The listing builds one solid part. Answer for the finished solid, in the listing's coordinates (mm). A direction names the side the tool comes from. Round coordinates to 2 decimals unless told otherwise and drop trailing zeros. Loops run counter-clockwise (first coordinate to the right, second up) from the corner with the lowest first, then second, coordinate; pieces in that order, holes last. Notation, with made-up numbers: M 55.5,54 L 64.5,54 A22 cw 64.5,69 Z; hole C 13.25,-0.75 d4. An arc over 180 degrees is marked long. Put each result on its own line as item: value. Start each with the question number.
(1) Which of the six approach directions +Z, -Z, +X, -X, +Y, -Y give full straight-line access (tool end or side, diameter ignored) to faces 1 (the face through (4.568, -7.924, 0.066)), 2 (the face through (2.958, -9.36, 2.726)), 3 (the face through (2.96, 8.5, 4.72)), 4 (the face through (2.958, -8.994, 3.703))?
(2) Straight lines are drawn through the part: line 1 (X direction, y = -5.5, z = -3.25); line 2 (Y direction, x = 0.7, z = 0); line 3 (Y direction, x = 4.75, z = -3.25). For each, find the intervals that lie inside material, in ascending order.
(3) Flat-ended cylindrical pins translate along their axes: P1, Ø3, axis at x = 2.5, y = 4.5, coming from the +Z side; P2, Ø1.6, axis at x = 4, z = -5.5, coming from the -Y side; P3, Ø1.2, axis at x = 5, y = -6, coming from the -Z side; P4, Ø11.5, axis at y = 0, z = 0, coming from the -X side. Find the tip coordinate at first contact, or state that the pin passes through.
(4) Determine the mould class of faces 5 (the face through (3, 5.6, 7.9)), 6 (the face through (2.96, 4.74, 8.52)), 7 (the face through (0, 0, 5)) for opening direction Z: released by +Z, released by -Z, zero draft, split by the parting line, or undercut.
(5) Section A-A, the plane z = 0 is taken. Determine the outline of the cut face in (x, y).
```python
from build123d import *
from build123d.topology import SkipClean

# Parameters (mm, degrees)
BASPROSKE_W                     = 6
BASPROSKE_H                     = 10.5
TOOTHCUT_DEPTH                  = 17.015617378
TEETHCUTS_COUNT                 = 28
TEETHCUTS_ANGLE                 = 347.142857143
BORSKE_R                        = 1.5
BORE_DEPTH                      = 50.0000508
SZKIC1_R                        = 6.75
WYTNIJ_WYCI_GNI_CIE1_DEPTH      = 2.7
SZKIC2_R                        = 4.5
WYTNIJ_WYCI_GNI_CIE2_DEPTH      = 16.148783562
SZKIC3_W                        = 8.9
SZKIC3_H                        = 2.106468257
SZKIC3_W_2                      = 2.106468257
SZKIC3_H_2                      = 8.9
WYTNIJ_WYCI_GNI_CIE3_DEPTH      = 2.7
WYTNIJ_WYCI_GNI_CIE4_DEPTH      = 16.148783562
WYTNIJ_WYCI_GNI_CIE4_DEPTH_BACK = 16.148783562
SFAZOWANIE1_SIZE                = 0.2
SFAZOWANIE2_SIZE                = 0.5


with BuildPart() as part:
    # BasProSke → Base-Revolve (revolve)
    with BuildSketch(Plane(origin=(0, 0, 0), x_dir=(1, 0, 0), z_dir=(0, 1, 0)), mode=Mode.PRIVATE) as base_revolve_sk:
        with Locations((3, 5.25)):
            Rectangle(BASPROSKE_W, BASPROSKE_H)
    revolve(base_revolve_sk.sketch.rotate(Axis((-10, 0, 0), (1, 0, 0)), 180), axis=Axis((-10, 0, 0), (1, 0, 0)))

    # TooCutSke → ToothCut (cut, through all)
    with BuildSketch(Plane(origin=(0, 0, 0), x_dir=(0, 0, -1), z_dir=(1, 0, 0))):
        with BuildLine():
            ThreePointArc((0.330517784, 8.917877213), (0, 8.924), (-0.330517784, 8.917877213))
            ThreePointArc((-0.330517784, 8.917877213), (-0.576240803, 9.73440515), (-0.992712377, 10.478481154))
            ThreePointArc((-0.992712377, 10.478481154), (0, 10.5254), (0.992712377, 10.478481154))
            ThreePointArc((0.992712377, 10.478481154), (0.576240803, 9.73440515), (0.330517784, 8.917877213))
        make_face()
    toothcut = extrude(amount=TOOTHCUT_DEPTH, mode=Mode.SUBTRACT)

    # TeethCuts: ToothCut ×28 about axis
    teethcuts_axis = Axis((-10, 0, 0), (1, 0, 0))
    for i in range(1, TEETHCUTS_COUNT):
        add(toothcut.rotate(teethcuts_axis, i * TEETHCUTS_ANGLE / (TEETHCUTS_COUNT - 1)), mode=Mode.SUBTRACT)

    # BorSke → Bore (cut, symmetric)
    with BuildSketch(Plane(origin=(0, 0, 0), x_dir=(0, 0, -1), z_dir=(1, 0, 0))):
        with Locations(Location((0, 0, 0), (0, 0, 180))):
            Circle(BORSKE_R)
    extrude(amount=BORE_DEPTH, both=True, mode=Mode.SUBTRACT)

    # Szkic1 → Wytnij-wyciągnięcie1 (cut)
    with BuildSketch(Plane(origin=(6, 0, 0), x_dir=(0, 0, -1), z_dir=(1, 0, 0))):
        Circle(SZKIC1_R)
    extrude(amount=-WYTNIJ_WYCI_GNI_CIE1_DEPTH, mode=Mode.SUBTRACT)

    # Szkic2 → Wytnij-wyciągnięcie2 (cut, through all)
    with BuildSketch(Plane(origin=(3.3, 0, 0), x_dir=(0, 0, -1), z_dir=(1, 0, 0))):
        Circle(SZKIC2_R)
    extrude(amount=-WYTNIJ_WYCI_GNI_CIE2_DEPTH, mode=Mode.SUBTRACT)

    # Szkic3 → Wytnij-wyciągnięcie3 (cut)
    with BuildSketch(Plane(origin=(6, 0, 0), x_dir=(0, 0, -1), z_dir=(1, 0, 0))):
        with Locations((0, 5.503234129)):
            Rectangle(SZKIC3_W, SZKIC3_H)
        with Locations((-5.503234129, 0)):
            Rectangle(SZKIC3_W_2, SZKIC3_H_2)
        with BuildLine():
            ThreePointArc((-6.556468257, 4.45), (-7.924, 0), (-6.556468257, -4.45))
            Line((-6.556468257, -4.45), (-6.556468257, 4.45))
        make_face()
        with BuildLine():
            Line((-4.45, 6.556468257), (4.45, 6.556468257))
            ThreePointArc((4.45, 6.556468257), (0, 7.924), (-4.45, 6.556468257))
        make_face()
        with BuildLine():
            Line((6.556468257, 4.45), (6.556468257, -4.45))
            ThreePointArc((6.556468257, -4.45), (7.574405273, -2.327694303), (7.924, 0))
            ThreePointArc((7.924, 0), (7.574405273, 2.327694303), (6.556468257, 4.45))
        make_face()
        with Locations((5.503234129, 0)):
            Rectangle(SZKIC3_W_2, SZKIC3_H_2)
        with BuildLine():
            ThreePointArc((-4.45, -6.556468257), (0, -7.924), (4.45, -6.556468257))
            Line((4.45, -6.556468257), (-4.45, -6.556468257))
        make_face()
        with Locations((0, -5.503234129)):
            Rectangle(SZKIC3_W, SZKIC3_H)
    extrude(amount=-WYTNIJ_WYCI_GNI_CIE3_DEPTH, mode=Mode.SUBTRACT)

    # Szkic4 → Wytnij-wyciągnięcie4 (cut, two sides: drawn at the far end of the back side and taken through both)
    with SkipClean():  # the faces are left unmerged after this step: merging them gives an invalid solid
        with BuildSketch(Plane(origin=(3.3, 0, 0), x_dir=(0, 0, -1), z_dir=(1, 0, 0)).offset(-WYTNIJ_WYCI_GNI_CIE4_DEPTH_BACK)):
            with BuildLine():
                Line((0, 10.924), (0, 8.924))
                ThreePointArc((0, 8.924), (8.924, 0), (0, -8.924))
                Line((0, -8.924), (0, -10.924))
                ThreePointArc((0, -10.924), (10.924, 0), (0, 10.924))
            make_face()
        extrude(amount=WYTNIJ_WYCI_GNI_CIE4_DEPTH + WYTNIJ_WYCI_GNI_CIE4_DEPTH_BACK, mode=Mode.SUBTRACT)

    # Sfazowanie1
    sfazowanie1_edges = [part.edges().sort_by_distance(p)[0] for p in [
        (6, 4.772970773, -4.772970773),
        (6, -4.772970773, 4.772970773),
        (6, 4.45, 5.815949636),
        (6, 0, 7.924),
        (6, -4.45, 5.815949636),
        (6, 4.45, -5.815949636),
        (6, 0, -7.924),
        (6, -4.45, -5.815949636),
        (6, 4.772970773, 4.772970773),
        (6, 5.815949636, -4.45),
        (6, 7.924, 0),
        (6, 5.815949636, 4.45),
        (6, -4.772970773, -4.772970773),
        (6, -5.815949636, -4.45),
        (6, -7.924, 0),
        (6, -5.815949636, 4.45),
    ]]
    chamfer(sfazowanie1_edges, length=SFAZOWANIE1_SIZE)

    # Sfazowanie2
    sfazowanie2_edges = [part.edges().sort_by_distance(p)[0] for p in [
        (3.3, 0, 4.5),
    ]]
    chamfer(sfazowanie2_edges, length=SFAZOWANIE2_SIZE)


solid = part.part
```
Recorded:
1. face 1: +X
1. face 2: +X, -X, -Y
1. face 3: +X, -X, +Y
1. face 4: +X, -X
2. line 1: x = 0 to 3.3
2. line 2: y = -8.92 to -4.5, 4.5 to 8.92
2. line 3: y = -8.31 to -7.23, 7.23 to 8.31
3. P1: stops at z = 9.98
3. P2: stops at y = -7.59
3. P3: stops at z = -7.1
3. P4: stops at x = 0
4. face 5: undercut
4. face 6: released by +Z
4. face 7: zero draft
5. outline: M 0,-8.92 L 6,-8.92 L 6,-8.12 L 5.8,-7.92 L 3.3,-7.92 L 3.3,-5 L 2.8,-4.5 L 0,-4.5 Z; M 0,4.5 L 2.8,4.5 L 3.3,5 L 3.3,7.92 L 5.8,7.92 L 6,8.12 L 6,8.92 L 0,8.92 Z
